```python
from build123d import *

# Parameters (mm, degrees)
SKETCH1_R           = 6.35
BOSS_EXTRUDE1_DEPTH = 1.6002


with BuildPart() as part:
    # Sketch1 → Boss-Extrude1 (new body)
    with BuildSketch(Plane.XY):
        with BuildLine():
            Line((-25.191875828, 0), (-25.191875828, -35.215356132))
            ThreePointArc((-25.191875828, -35.215356132), (-25.144594979, -35.781140778), (-25.004063999, -36.331230578))
            add(Edge.make_bspline(
                [(-25.004063999, -36.331230578), (-24.302161584, -38.357321078), (-17.500345693, -49.472928078), (6.486565439, -52.353017034), (16.828257208, -40.890808587), (18.117618202, -36.640731795)],
                knots=[0.011286064, 0.011286064, 0.011286064, 0.011286064, 0.130987572, 0.750185474, 0.983991621, 0.983991621, 0.983991621, 0.983991621], degree=3))
            ThreePointArc((18.117618202, -36.640731795), (18.258374718, -35.854153527), (18.212152653, -35.056418427))
            add(Edge.make_bspline(
                [(18.212152653, -35.056418427), (15.722327617, -21.003254002), (45.083704914, -12.577387864), (50.314621311, -12.487786805)],
                knots=[0.243688719, 0.243688719, 0.243688719, 0.243688719, 1, 1, 1, 1], degree=3))
            add(Edge.make_bspline(
                [(50.314621311, -12.487786805), (67.828969762, -11.217353563), (162.851239243, 6.097445829), (250.038282618, -9.041784468), (279.934807735, -2.602592093)],
                knots=[0.23584572, 0.23584572, 0.23584572, 0.23584572, 0.495200792, 0.941477437, 0.941477437, 0.941477437, 0.941477437], degree=3))
            ThreePointArc((279.934807735, -2.602592093), (281.939894054, -0.09633433), (279.889362488, 2.372880002))
            add(Edge.make_bspline(
                [(2.090204907, 25.105012471), (29.372633882, 21.318909318), (128.041674084, 14.540572725), (239.548411309, 10.293455518), (279.889362488, 2.372880002)],
                knots=[0.008543469, 0.008543469, 0.008543469, 0.008543469, 0.340594684, 0.94139515, 0.94139515, 0.94139515, 0.94139515], degree=3))
            ThreePointArc((2.090204907, 25.105012471), (-17.058347301, 18.537621075), (-25.191875828, 0))
        make_face()
        with Locations((0, -25.4)):
            Circle(SKETCH1_R, mode=Mode.SUBTRACT)
        Circle(SKETCH1_R, mode=Mode.SUBTRACT)
    extrude(amount=BOSS_EXTRUDE1_DEPTH)


solid = part.part
```
Work out the finished part from the listing and answer in its coordinate system (mm). Round coordinates to 2 decimals unless told otherwise and drop trailing zeros. Write each question's results on one line, items separated by ' | '.
1) A flat-ended cylindrical pin translates along its axis: pin 1 (10 mm diameter, centred on x = 0, y = -25.4, fed in from -Z). Find the tip coordinate at first contact, or state that the pin passes through.
Findings:
pin 1: passes through
2) For a pull along Y with two mould halves and no side action, classify faces 1 (the flat face through (71, -5, 0)), 2 (the cylindrical face through (-1.38, -6.2, 0.79)), 3 (the cylindrical face through (-1.38, -31.6, 0.79)), 4 (the cylindrical face through (-16.843, 18.734, 0.789)) as +Y half, -Y half, draft (parallel to the pull), parting line (faces both ways), or undercut.
Findings:
face 1: draft | face 2: undercut | face 3: undercut | face 4: +Y half
3) Consider line 1 along Y through (x, z) = (0, 0.65); line 2 along X through (y, z) = (2, 1.4); line 3 along Y through (x, z) = (50.5, 0.7). Determine where each line is inside the solid, lowest interval first. Write a range as [from, to].
Findings:
line 1: y = [-49.2, -31.75], [-19.05, -6.35], [6.35, 25.19] | line 2: x = [-25.11, -6.03], [6.03, 280.8] | line 3: y = [-12.47, 20.14]
4) The part is cut by section A-A (x = -2). State how many separate pieces and enclosed holes the cut face has, and give its area (3 significant figures).
Findings:
separate pieces: 3 | enclosed holes: 0 | area: 80.5 mm²
